Check sheet for the modelled part. Datum: model origin and axes. Units: mm. Face numbers are marked on the shaded views. A direction names the side the tool comes from. Round coordinates to 2 decimals unless told otherwise and drop trailing zeros. Order: outer loops, then holes, each group sorted by start corner. A loop starts at its lowest first (then second) coordinate and runs counter-clockwise, first axis right, second up.
Q1. Scan lines: probe 1 along X at (y, z) = (2.4, 0); probe 2 along X at (y, z) = (1, 0); probe 3 along Z at (x, y) = (4.5, 2.2). Record each from-to range of solid material in increasing order.
Q2. Cross-section at B-B on z = -10. Record the cut outline in (x, y), then the cut area to 3 significant figures.
Q3. Set-up check for the marked faces 1, 2 and 3: record each of +Z, -Z, +X, -X, +Y, -Y from which the full face is reachable in a straight line by a thin tool's end or side.
Q4. Cross-section at C-C on y = 0.7. Record the cut outline in (x, z).
Q5. Depth check by flat-ended pin: P1, Ø1.2, axis at x = 10.5, z = 0, coming from the +Y side; P2, Ø0.9, axis at y = 1.5, z = -11.5, coming from the +X side; P3, Ø0.9, axis at y = 1, z = -10, coming from the -X side. Enter the tip coordinate at first touch or a pass-through.
Q6. Cross-section at A-A on x = 10. Record the cut outline in (y, z).
Q7. Cross-section at D-D on z = 0. Record the cut outline in (x, y), then the cut area to 3 significant figures.
from build123d import *

# Parameters (mm, degrees)
SKETCH1_W           = 11.5
SKETCH1_H           = 7
SKETCH1_R           = 2
SKETCH1_W_2         = 7
SKETCH1_H_2         = 11.5
SKETCH1_R_2         = 1
BOSS_EXTRUDE1_DEPTH = 3
SKETCH1_3_R         = 2
SKETCH1_3_R_2       = 1
BOSS_EXTRUDE2_DEPTH = 2


with BuildPart() as part:
    # Sketch1 → Boss-Extrude1 (new body)
    with BuildSketch(Plane(origin=(0, 0, 0), x_dir=(1, 0, 0), z_dir=(0, 1, 0))):
        with Locations((-9.25, 0)):
            Rectangle(SKETCH1_W, SKETCH1_H)
        with Locations((-10, 0)):
            Circle(SKETCH1_R, mode=Mode.SUBTRACT)
        Rectangle(SKETCH1_W_2, SKETCH1_H)
        with Locations((9.25, 0)):
            Rectangle(SKETCH1_W, SKETCH1_H)
        with Locations((10, 0)):
            Circle(SKETCH1_R, mode=Mode.SUBTRACT)
        with Locations((0, 9.25)):
            Rectangle(SKETCH1_W_2, SKETCH1_H_2)
        with Locations((0, 10)):
            Circle(SKETCH1_R, mode=Mode.SUBTRACT)
        with Locations((0, -9.25)):
            Rectangle(SKETCH1_W_2, SKETCH1_H_2)
        with Locations((0, -10)):
            Circle(SKETCH1_R, mode=Mode.SUBTRACT)
        with Locations((0, 10)):
            Circle(SKETCH1_R)
        with Locations((0, 10)):
            Circle(SKETCH1_R_2, mode=Mode.SUBTRACT)
        with Locations((0, -10)):
            Circle(SKETCH1_R)
        with Locations((0, -10)):
            Circle(SKETCH1_R_2, mode=Mode.SUBTRACT)
    extrude(amount=BOSS_EXTRUDE1_DEPTH)

    # Sketch1_3 → Boss-Extrude2 (add)
    with BuildSketch(Plane(origin=(0, 0, 0), x_dir=(1, 0, 0), z_dir=(0, 1, 0))):
        with Locations((-10, 0)):
            Circle(SKETCH1_3_R)
        with Locations((-10, 0)):
            Circle(SKETCH1_3_R_2, mode=Mode.SUBTRACT)
        with Locations((10, 0)):
            Circle(SKETCH1_3_R)
        with Locations((10, 0)):
            Circle(SKETCH1_3_R_2, mode=Mode.SUBTRACT)
    extrude(amount=BOSS_EXTRUDE2_DEPTH)


solid = part.part
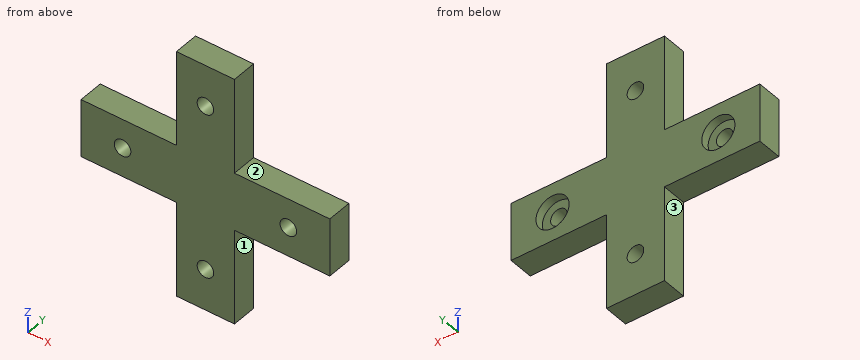
Results found:
1. probe 1: x = -15 to -12, -8 to 8, 12 to 15
1. probe 2: x = -15 to -11, -9 to 9, 11 to 15
1. probe 3: z = -3.5 to 3.5
2. outline: (-3.5, 0) - (-1, 0) - (-1, 3) - (-3.5, 3) - close; (1, 0) - (3.5, 0) - (3.5, 3) - (1, 3) - close
2. area: 15.0 mm2
3. face 1: -Z, +X, +Y, -Y
3. face 2: +Z, +X, +Y, -Y
3. face 3: -Z, -X, +Y, -Y
4. outline: (-15, -3.5) - (-3.5, -3.5) - (-3.5, -15) - (3.5, -15) - (3.5, -3.5) - (15, -3.5) - (15, 3.5) - (3.5, 3.5) - (3.5, 15) - (-3.5, 15) - (-3.5, 3.5) - (-15, 3.5) - close; hole circle Ø2 at (-10, 0); hole circle Ø2 at (0, -10); hole circle Ø2 at (0, 10); hole circle Ø2 at (10, 0)
5. P1: stops at y = 2
5. P2: stops at x = 3.5
5. P3: stops at x = -3.5
6. outline: (0, -3.5) - (3, -3.5) - (3, -2) - (2, -2) - (2, -1) - (0, -1) - close; (0, 1) - (2, 1) - (2, 2) - (3, 2) - (3, 3.5) - (0, 3.5) - close
7. outline: (-15, 0) - (-11, 0) - (-11, 2) - (-12, 2) - (-12, 3) - (-15, 3) - close; (-9, 0) - (9, 0) - (9, 2) - (8, 2) - (8, 3) - (-8, 3) - (-8, 2) - (-9, 2) - close; (11, 0) - (15, 0) - (15, 3) - (12, 3) - (12, 2) - (11, 2) - close
7. area: 74.0 mm2
